Verification items for this drawing (mm, ordinates from the low corner). A direction names the side the tool comes from. Round coordinates to 2 decimals unless told otherwise and drop trailing zeros. Order: outer loops, then holes, each group sorted by start corner. A loop starts at its lowest first (then second) coordinate and runs counter-clockwise, first axis right, second up. Notation, with made-up numbers: (2, 48.5) -> (13, 48.5) arc R13 ccw to (13, 69.5) -> close; hole circle Ø5 at (-3.5, 38.5). An arc over 180 degrees is marked (long way). Use a Markdown table: item, result. Add a question column.
Item 1: Sectioned sample at B-B, the plane z = 15. Record the cut outline in (x, y), and give its area (3 significant figures).
Item 2: Sectioned sample at C-C, the plane x = 3.5. Record the cut outline in (y, z).
Item 3: Gauge pin test, flat ends, axial feed: pin 1 Ø8 at (x, z) = (10.5, 33.5) entering from -Y; pin 2 Ø16 at (y, z) = (23, 23.5) entering from -X. Record the tip position at first contact, or that the pin passes through.
Item 4: Set-up check for the marked faces 1 and 2: record each of +Z, -Z, +X, -X, +Y, -Y from which the full face is reachable in a straight line by a thin tool's end or side.
Item 5: Sectioned sample at A-A, the plane z = 38.5. Record the cut outline in (x, y), and give its area (3 significant figures).
Item 6: Material ranges on probe 1 along X at (y, z) = (36, 38.95); probe 2 along Y at (x, z) = (5, 6.5), recorded low to high. Write a range as [from, to].
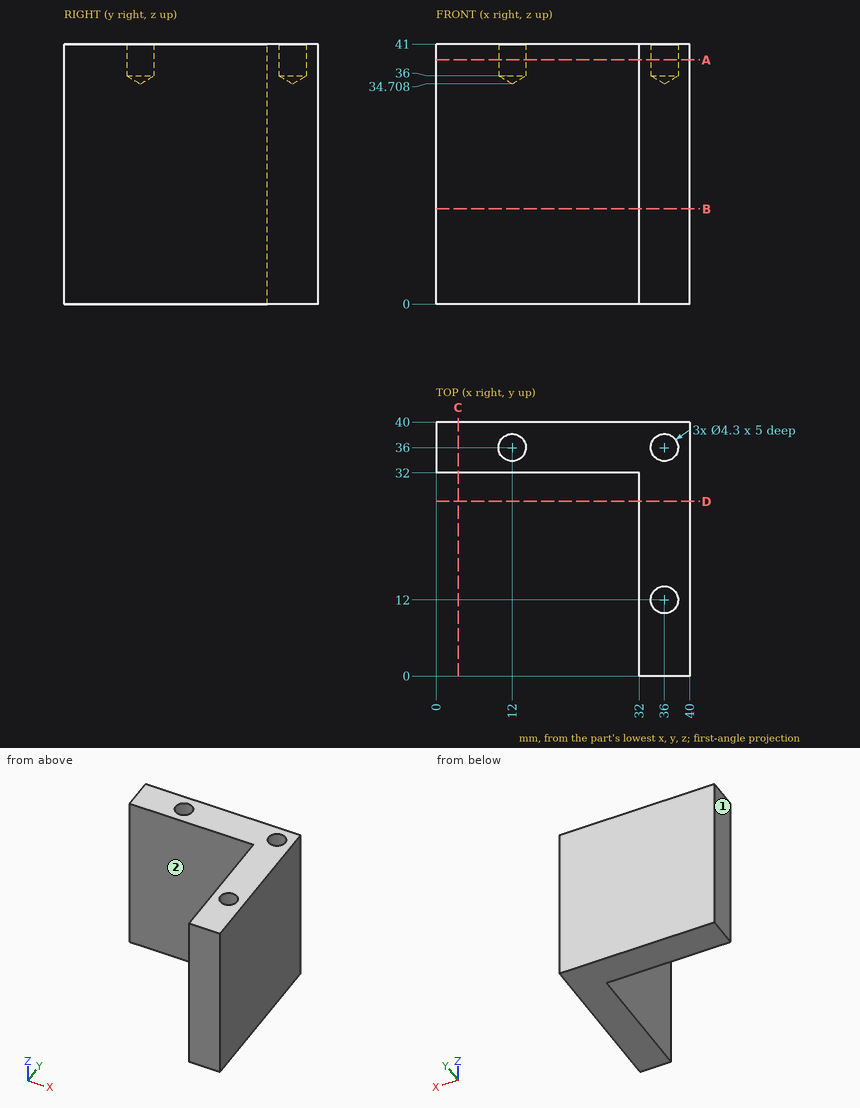
Found:
| question | item | result |
|---|---|---|
| 1 | outline | (0, 32) -> (32, 32) -> (32, 0) -> (40, 0) -> (40, 40) -> (0, 40) -> close |
| 1 | area | 576 mm2 |
| 2 | outline | (32, 0) -> (40, 0) -> (40, 41) -> (32, 41) -> close |
| 3 | pin 1 | stops at y = 32 |
| 3 | pin 2 | stops at x = 32 |
| 4 | face 1 | +Z, -Z, -X, +Y, -Y |
| 4 | face 2 | +Z, -Z, -X, -Y |
| 5 | outline | (0, 32) -> (32, 32) -> (32, 0) -> (40, 0) -> (40, 40) -> (0, 40) -> close; hole circle Ø4.3 at (12, 36); hole circle Ø4.3 at (36, 12); hole circle Ø4.3 at (36, 36) |
| 5 | area | 532 mm2 |
| 6 | probe 1 | x = [0, 9.85], [14.15, 33.85], [38.15, 40] |
| 6 | probe 2 | y = [32, 40] |
